CAD build for the part. Positions are in the model's coordinates, mm. Give positions to 0.01 mm unless a question says otherwise; leave off trailing zeros. Write each loop counter-clockwise with the first axis right and the second up, starting at its lowest first coordinate (ties: lowest second). Pieces come first, ordered by that corner, then holes. Notation, with made-up numbers: (6, 55) - (24, 55) arc R19 cw to (24, 82) - close; hole circle Ø1 at (-26, 42). An arc over 180 degrees is marked (long way). Answer as a JSON object with one key per item and string values.
Autodesk Inventor part; units mm, degrees
ref_plane "YZ Plane" through (0, 0, 0) normal (1, 0, 0) x (0, 1, 0)
ref_plane "XZ Plane" through (0, 0, 0) normal (0, 1, 0) x (-1, 0, 0)
ref_plane "XY Plane" through (0, 0, 0) normal (0, 0, 1) x (1, 0, 0)
sketch "Schizzo1" plane through (0, 0, 0) normal (0, 0, 1) x (1, 0, 0)
  line L0 (0, 0) -> (22.7, 0)
  line L1 (22.7, 0) -> (22.7, 7)
  line L2 (22.7, 7) -> (0, 7)
  line L3 (0, 7) -> (0, 0)
  dimension "d0" = 22.7
  dimension "d2" = 7
extrude "Estrusione1" add sketch "Schizzo1" along normal blind 1.3
sketch "Sketch2" plane through (0, 0, 1.3) normal (0, 0, 1) x (1, 0, 0)
  line L0 (6.85, 4) -> (16.85, 4)
  line L1 (16.85, 4) -> (16.85, 2.5)
  line L2 (16.85, 2.5) -> (6.85, 2.5)
  line L3 (6.85, 2.5) -> (6.85, 4)
  line L4 (0, 7) -> (0, 0)
  line L5 (0, 0) -> (22.7, 0)
  point P0 (0, 6.5)
  dimension "d6" = 10
  dimension "d7" = 1.5
  dimension "d8" = 6.85
  dimension "d9" = 2.5
extrude "Handle" add sketch "Sketch2" along normal blind 1
fillet "Fillet2" radius 0.5 8 edges at (16.85, 4, 1.8) (16.85, 2.5, 1.8) (6.85, 4, 1.8) (6.85, 2.5, 1.8) (11.85, 2.5, 2.3) (16.85, 3.25, 2.3) (6.85, 3.25, 2.3) (11.85, 4, 2.3)
fillet "Fillet3" radius 0.6 8 edges at (0, 7, 0.65) (22.7, 7, 0.65) (0, 3.5, 1.3) (0, 3.5, 0) (22.7, 3.5, 1.3) (22.7, 3.5, 0) (11.35, 7, 1.3) (11.35, 7, 0)
properties part number "160409 T-RH-P Box cap R23p"
Item 1: Cut at B-B (z = 2.1). Give the cut face in (x, y), and give its area (3 significant figures).
Entries:
{"outline": "(6.95, 3) arc R0.4 ccw to (7.35, 2.6) - (16.35, 2.6) arc R0.4 ccw to (16.75, 3) - (16.75, 3.5) arc R0.4 ccw to (16.35, 3.9) - (7.35, 3.9) arc R0.4 ccw to (6.95, 3.5) - close", "area": "12.6 mm2"}
Item 2: Cut at D-D (x = 14.75). Give the cut face in (y, z), and give its area (3 significant figures).
Entries:
{"outline": "(0, 0) - (6.4, 0) arc R0.6 ccw to (7, 0.6) - (7, 0.7) arc R0.6 ccw to (6.4, 1.3) - (4, 1.3) - (4, 1.8) arc R0.5 ccw to (3.5, 2.3) - (3, 2.3) arc R0.5 ccw to (2.5, 1.8) - (2.5, 1.3) - (0, 1.3) - close", "area": "10.3 mm2"}
Item 3: Cut at A-A (x = 19.5). Give the cut face in (y, z).
Entries:
{"outline": "(0, 0) - (6.4, 0) arc R0.6 ccw to (7, 0.6) - (7, 0.7) arc R0.6 ccw to (6.4, 1.3) - (0, 1.3) - close"}
Item 4: Probe line 1 (Z direction, x = 1.25, y = 4.25); line 2 (X direction, y = 3.5, z = 1.6); line 3 (Y direction, x = 15.75, z = 1.7). List the from-to ranges inside material, lowest first. Write a range as from..to.
Entries:
{"line 1": "0..1.3", "line 2": "6.85..16.85", "line 3": "2.5..4"}
Item 5: Cut at C-C (y = 2). Give the cut face in (x, z).
Entries:
{"outline": "(0, 0.6) arc R0.6 ccw to (0.6, 0) - (22.1, 0) arc R0.6 ccw to (22.7, 0.6) - (22.7, 0.7) arc R0.6 ccw to (22.1, 1.3) - (0.6, 1.3) arc R0.6 ccw to (0, 0.7) - close"}
